```python
from build123d import *

# Parameters (mm, degrees)
F1_DEPTH = 30
F2_W     = 5.75
F2_H     = 23
F3_DEPTH = 4
F2_W_2   = 4.2
F2_H_2   = 4
F2_H_3   = 6
F4_DEPTH = 4


with BuildPart() as f1:
    # F0 (on Front) → F1 (new body)
    with BuildSketch(Plane.XZ):
        Polygon((0, 4), (0, 0), (50.75, 0), (50.75, 3.25), (50.75, 4), (50.15, 4), (50.15, 3.25), (48.744, 3.25), (48.744, 4), (48.144, 4), (48.144, 3.25), (46.738, 3.25), (46.738, 4), (46.138, 4), (46.138, 3.25), (44.732, 3.25), (44.732, 4), (44.132, 4), (44.132, 3.25), (42.726, 3.25), (42.726, 4), (42.126, 4), (42.126, 3.25), (40.72, 3.25), (40.72, 4), (40.12, 4), (40.12, 3.25), (38.714, 3.25), (38.714, 4), (38.114, 4), (38.114, 3.25), (36.708, 3.25), (36.708, 4), (36.108, 4), (36.108, 3.25), (34.702, 3.25), (34.702, 4), (34.102, 4), (34.102, 3.25), (32.696, 3.25), (32.696, 4), (32.096, 4), (32.096, 3.25), (30.69, 3.25), (30.69, 4), (30.09, 4), (30.09, 3.25), (28.684, 3.25), (28.684, 4), (28.084, 4), (28.084, 3.25), (26.678, 3.25), (26.678, 4), (26.078, 4), (26.078, 3.25), (24.672, 3.25), (24.672, 4), (24.072, 4), (24.072, 3.25), (22.666, 3.25), (22.666, 4), (22.066, 4), (22.066, 3.25), (20.66, 3.25), (20.66, 4), (20.06, 4), (20.06, 3.25), (18.654, 3.25), (18.654, 4), (18.054, 4), (18.054, 3.25), (16.648, 3.25), (16.648, 4), (16.048, 4), (16.048, 3.25), (14.642, 3.25), (14.642, 4), (14.042, 4), (14.042, 3.25), (12.636, 3.25), (12.636, 4), (12.036, 4), (12.036, 3.25), (10.63, 3.25), (10.63, 4), (10.03, 4), (10.03, 3.25), (8.624, 3.25), (8.624, 4), (8.324, 4), (8.024, 4), (8.024, 3.25), (6.618, 3.25), (6.618, 4), (6.318, 4), (6.018, 4), (6.018, 3.25), (4.612, 3.25), (4.612, 4), (4.012, 4), (4.012, 3.25), (2.606, 3.25), (2.606, 4), (2.006, 4), (2.006, 3.25), (0.6, 3.25), (0.6, 4), align=None)
    extrude(amount=F1_DEPTH)

    # F2 (on face) → F3 (cut, through all)
    with BuildSketch(Plane(origin=(0, 0, 0), x_dir=(1, 0, 0), z_dir=(0, 0, -1))):
        with Locations((22.5, 18.5)):
            Rectangle(F2_W, F2_H)
        with Locations((28.25, 18.5)):
            Rectangle(F2_W, F2_H)
    extrude(amount=-F3_DEPTH, mode=Mode.SUBTRACT)

    # F2 (on face) → F4 (cut, through all)
    with BuildSketch(Plane(origin=(0, 0, 0), x_dir=(1, 0, 0), z_dir=(0, 0, -1))):
        with BuildLine():
            ThreePointArc((12.375, 8.55227), (10.275, 10.65227), (8.175, 8.55227))
            Line((8.175, 8.55227), (12.375, 8.55227))
        make_face()
        with Locations((10.275, 6.55227)):
            Rectangle(F2_W_2, F2_H_2)
        with BuildLine():
            Line((12.375, 4.55227), (8.175, 4.55227))
            ThreePointArc((8.175, 4.55227), (10.275, 2.45227), (12.375, 4.55227))
        make_face()
        with BuildLine():
            ThreePointArc((42.525, 8.55227), (40.425, 10.65227), (38.325, 8.55227))
            Line((38.325, 8.55227), (42.525, 8.55227))
        make_face()
        with Locations((40.425, 6.55227)):
            Rectangle(F2_W_2, F2_H_2)
        with BuildLine():
            Line((42.525, 4.55227), (38.325, 4.55227))
            ThreePointArc((38.325, 4.55227), (40.425, 2.45227), (42.525, 4.55227))
        make_face()
        with BuildLine():
            ThreePointArc((10.575, 26.55227), (8.475, 28.65227), (6.375, 26.55227))
            Line((6.375, 26.55227), (10.575, 26.55227))
        make_face()
        with Locations((8.475, 24.55227)):
            Rectangle(F2_W_2, F2_H_2)
        with BuildLine():
            Line((10.575, 22.55227), (6.375, 22.55227))
            ThreePointArc((6.375, 22.55227), (8.475, 20.45227), (10.575, 22.55227))
        make_face()
        with BuildLine():
            ThreePointArc((45.075, 24.05227), (42.975, 26.15227), (40.875, 24.05227))
            Line((40.875, 24.05227), (45.075, 24.05227))
        make_face()
        with Locations((42.975, 21.05227)):
            Rectangle(F2_W_2, F2_H_3)
        with BuildLine():
            Line((45.075, 18.05227), (40.875, 18.05227))
            ThreePointArc((40.875, 18.05227), (42.975, 15.95227), (45.075, 18.05227))
        make_face()
    extrude(amount=-F4_DEPTH, mode=Mode.SUBTRACT)


solid = f1.part
```
The model under review builds one solid part; all positions refer to its coordinate system, in mm. A direction names the side the tool comes from. Round coordinates to 2 decimals unless told otherwise and drop trailing zeros. Order: outer loops, then holes, each group sorted by start corner. A loop starts at its lowest first (then second) coordinate and runs counter-clockwise, first axis right, second up. Notation, with made-up numbers: (8, -16.75) - (41, -16.75) arc R21 cw to (41, 19.25) - close; hole circle Ø1 at (11.5, 14). An arc over 180 degrees is marked (long way). Answer in a Markdown table with one row per item.
(1) For line 1 (X direction, y = -19.5, z = 1.8) (3 decimals); line 2 (X direction, y = -16.5, z = 2.3) (3 decimals); line 3 (X direction, y = -15, z = 2.55) (3 decimals), list the stretches that pass through material, from the lowest coordinate up. Write a range as from..to.
Result set:
| item | result |
|---|---|
| line 1 | x = 0..19.625, 31.125..40.875, 45.075..50.75 |
| line 2 | x = 0..19.625, 31.125..41.561, 44.389..50.75 |
| line 3 | x = 0..19.625, 31.125..50.75 |
(2) Clearance check with a flat-ended pin moving along its axis: P1, Ø0.7, axis at x = 39.5, y = -2, coming from the +Z side. State where the tip first meets the part, or that it passes through.
Result set:
| item | result |
|---|---|
| P1 | stops at z = 3.25 |
(3) Take a section at B-B on z = 0.95. Write out the cut boundary in (x, y) (3 decimals), plus the area to 3 significant figures.
Result set:
| item | result |
|---|---|
| outline | (0, -30) - (19.625, -30) - (19.625, -7) - (31.125, -7) - (31.125, -30) - (50.75, -30) - (50.75, 0) - (0, 0) - close; hole (6.375, -26.552) arc R2.1 ccw to (10.575, -26.552) - (10.575, -22.552) arc R2.1 ccw to (6.375, -22.552) - close; hole (8.175, -8.552) arc R2.1 ccw to (12.375, -8.552) - (12.375, -4.552) arc R2.1 ccw to (8.175, -4.552) - close; hole (38.325, -8.552) arc R2.1 ccw to (42.525, -8.552) - (42.525, -4.552) arc R2.1 ccw to (38.325, -4.552) - close; hole (40.875, -24.052) arc R2.1 ccw to (45.075, -24.052) - (45.075, -18.052) arc R2.1 ccw to (40.875, -18.052) - close |
| area | 1,130 mm2 |
(4) Mouldability with a two-part tool opening along Y and no side actions: class faces 1 (the face through (39, -20, 3.25)), 2 (the face through (41, -30, 2)), 3 (the face through (45.075, -21, 2)) as released by +Y, released by -Y, zero draft, split by the parting line, or undercut.
Result set:
| item | result |
|---|---|
| face 1 | zero draft |
| face 2 | released by -Y |
| face 3 | undercut |
(5) Take a section at C-C on y = -7.75. Count the separate pieces of the cut face and the enclosed holes in it, plus the area to 3 significant figures.
Result set:
| item | result |
|---|---|
| separate pieces | 4 |
| enclosed holes | 0 |
| area | 107 mm2 |
(6) Machinability: for faces 4 (the face through (10.575, -25, 2)), 5 (the face through (31.125, -18, 2)), 6 (the face through (19, -15, 3.25)), which of the approach directions +Z, -Z, +X, -X, +Y, -Y give a long, thin tool a straight path to every point of the face, cutting with its end or side? Answer none if there is none.
Result set:
| item | result |
|---|---|
| face 4 | +Z, -Z |
| face 5 | +Z, -Z, -Y |
| face 6 | +Z, +Y, -Y |
(7) Take a section at A-A on x = 41.5. Write out the cut boundary in (y, z), plus the area to 3 significant figures.
Result set:
| item | result |
|---|---|
| outline | (-30, 0) - (-25.55, 0) - (-25.55, 3.25) - (-30, 3.25) - close; (-16.56, 0) - (-10.36, 0) - (-10.36, 3.25) - (-16.56, 3.25) - close; (-2.75, 0) - (0, 0) - (0, 3.25) - (-2.75, 3.25) - close |
| area | 43.6 mm2 |
